Model file for the job. Use its own axes, mm. Face numbers are marked on the shaded views. A direction names the side the tool comes from. Give positions to 0.01 mm unless a question says otherwise; leave off trailing zeros. Loops run counter-clockwise (first coordinate to the right, second up) from the corner with the lowest first, then second, coordinate; pieces in that order, holes last. Notation, with made-up numbers: M 56.5,80.5 L 110.5,80.5 A35 cw 110.5,113.5 Z; hole C 47,32.25 d10. An arc over 180 degrees is marked long. Answer in a Markdown table with one row per item.
```python
from build123d import *

# Parameters (mm, degrees)
CROQUIS1_R              = 1.25
SALIENTE_EXTRUIR1_DEPTH = 10
CROQUIS2_W              = 9
CROQUIS2_H              = 10
CORTAR_EXTRUIR1_DEPTH   = 4
CORTAR_EXTRUIR2_DEPTH   = 1.5
REDONDEO2_R             = 4


with BuildPart() as part:
    # Croquis1 → Saliente-Extruir1 (new body)
    with BuildSketch(Plane.XY):
        with BuildLine():
            Line((-68.837310195, 14.25), (-55.837310195, 14.25))
            Line((-55.837310195, 14.25), (-45.737310195, 24.35))
            Line((-45.737310195, 24.35), (-36.937310195, 24.35))
            Line((-36.937310195, 24.35), (-26.837310195, 14.25))
            Line((-26.837310195, 14.25), (-13.837310195, 14.25))
            Line((-13.837310195, 14.25), (-13.837310195, 4.25))
            Line((-13.837310195, 4.25), (-26.337310195, 4.25))
            ThreePointArc((-26.337310195, 4.25), (-41.337310195, 12.292271557), (-56.337310195, 4.25))
            Line((-56.337310195, 4.25), (-68.837310195, 4.25))
            Line((-68.837310195, 4.25), (-68.837310195, 14.25))
        make_face()
        with Locations((-18.087310195, 10.5)):
            Circle(CROQUIS1_R, mode=Mode.SUBTRACT)
        with Locations((-64.587310195, 10.5)):
            Circle(CROQUIS1_R, mode=Mode.SUBTRACT)
    extrude(amount=SALIENTE_EXTRUIR1_DEPTH)

    # Croquis2 → Cortar-Extruir1 (cut)
    with BuildSketch(Plane(origin=(0, 0, 0), x_dir=(-1, 0, 0), z_dir=(0, 0, -1))):
        with Locations((64.337310195, 9.25)):
            Rectangle(CROQUIS2_W, CROQUIS2_H)
        with Locations((18.337310195, 9.25)):
            Rectangle(CROQUIS2_W, CROQUIS2_H)
    extrude(amount=-CORTAR_EXTRUIR1_DEPTH, mode=Mode.SUBTRACT)

    # Croquis3 → Cortar-Extruir2 (cut)
    with BuildSketch(Plane(origin=(0, 0, 4), x_dir=(-1, 0, 0), z_dir=(0, 0, -1))):
        Polygon((62.104704038, 10.5), (63.346007116, 8.35), (65.828613274, 8.35), (67.069916353, 10.5), (65.828613274, 12.65), (63.346007116, 12.65), align=None)
        Polygon((15.604704038, 10.5), (16.846007116, 8.35), (19.328613274, 8.35), (20.569916353, 10.5), (19.328613274, 12.65), (16.846007116, 12.65), align=None)
    extrude(amount=-CORTAR_EXTRUIR2_DEPTH, mode=Mode.SUBTRACT)

    # Redondeo2
    redondeo2_edges = [part.edges().sort_by_distance(p)[0] for p in [
        (-68.837310195, 14.25, 7),
        (-45.737310195, 24.35, 5),
        (-36.937310195, 24.35, 5),
        (-13.837310195, 14.25, 7),
        (-13.837310195, 4.25, 7),
        (-26.337310195, 4.25, 5),
        (-56.337310195, 4.25, 5),
        (-68.837310195, 4.25, 7),
    ]]
    fillet(redondeo2_edges, radius=REDONDEO2_R)


solid = part.part
```
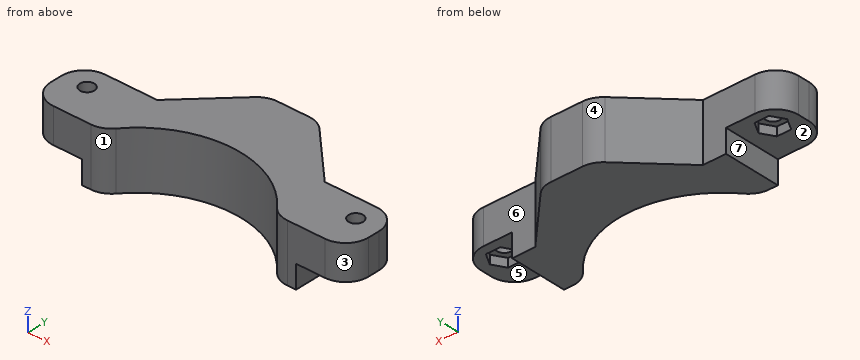
Q1. Saw through at D-D (y = 18). Give the cut face in (x, z), and give its area (3 significant figures).
Reported:
| item | result |
|---|---|
| outline | M -52.09,0 L -30.59,0 L -30.59,10 L -52.09,10 Z |
| area | 215 mm² |
Q2. Mould opens along X. For the marked faces 1, 2, 3 and 4 say: released by +X, released by -X, zero draft, split by the parting line, or undercut.
Reported:
| item | result |
|---|---|
| face 1 | undercut |
| face 2 | zero draft |
| face 3 | released by +X |
| face 4 | released by -X |
Q3. Drop flat-ended pins along their axis: pin 1 (4 mm diameter, centred on x = -38.5, z = 4, fed in from -Y); pin 2 (2 mm diameter, centred on y = 9.5, z = 2, fed in from +X); pin 3 (2.5 mm diameter, centred on x = -18.5, y = 9, fed in from -Z). Give the stop position or say it passes through.
Reported:
| item | result |
|---|---|
| pin 1 | y = 11.63 |
| pin 2 | x = -22.84 |
| pin 3 | z = 4 |
Q4. Probe probe 1 along X at (y, z) = (10.5, 7.5); probe 2 along Z at (x, y) = (-63.5, 5); probe 3 along Y at (x, z) = (-23, 5.75). List the from-to ranges inside material, lowest first.
Reported:
| item | result |
|---|---|
| probe 1 | -68.83 to -65.84, -63.34 to -49.17, -33.51 to -19.34, -16.84 to -13.85 |
| probe 2 | 4 to 10 |
| probe 3 | 4.25 to 14.25 |
Q5. Saw through at A-A (z = 8.25). Give the cut face in (x, y), and give its area (3 significant figures).
Reported:
| item | result |
|---|---|
| outline | M -68.84,8.25 A4 ccw -64.84,4.25 L -58.35,4.25 A4 ccw -55.26,5.71 A18.01 cw -27.42,5.71 A4 ccw -24.33,4.25 L -17.84,4.25 A4 ccw -13.84,8.25 L -13.84,10.25 A4 ccw -17.84,14.25 L -26.84,14.25 L -35.77,23.18 A4 ccw -38.59,24.35 L -44.08,24.35 A4 ccw -46.91,23.18 L -55.84,14.25 L -64.84,14.25 A4 ccw -68.84,10.25 Z; hole C -64.59,10.5 d2.5; hole C -18.09,10.5 d2.5 |
| area | 546 mm² |
Q6. 3-axis set-ups, long thin cutter, end or side, ignore diameter. For the marked faces 5, 6 and 7: which of +Z, -Z, +X, -X, +Y, -Y reach the whole face in a straight line?
Reported:
| item | result |
|---|---|
| face 5 | -Z, +X, +Y, -Y |
| face 6 | +Z, -Z, +X, +Y |
| face 7 | -Z, -X, +Y, -Y |
Q7. Saw through at C-C (x = -64). Give the cut face in (y, z).
Reported:
| item | result |
|---|---|
| outline | M 4.25,4 L 8.35,4 L 8.35,5.5 L 9.4,5.5 L 9.4,10 L 4.25,10 Z; M 11.6,5.5 L 12.65,5.5 L 12.65,4 L 14.25,4 L 14.25,10 L 11.6,10 Z |
Q8. Saw through at B-B (z = 0.5). Give the cut face in (x, y), and give its area (3 significant figures).
Reported:
| item | result |
|---|---|
| outline | M -59.84,4.25 L -58.35,4.25 A4 ccw -55.26,5.71 A18.01 cw -27.42,5.71 A4 ccw -24.33,4.25 L -22.84,4.25 L -22.84,14.25 L -26.84,14.25 L -35.77,23.18 A4 ccw -38.59,24.35 L -44.08,24.35 A4 ccw -46.91,23.18 L -55.84,14.25 L -59.84,14.25 Z |
| area | 389 mm² |
